Geometry: final body of the model. Coordinates: model frame, mm. A direction names the side the tool comes from. Coordinates: 2 decimals unless noted, no trailing zeros. Write each loop counter-clockwise with the first axis right and the second up, starting at its lowest first coordinate (ties: lowest second). Pieces come first, ordered by that corner, then holes. Notation, with made-up numbers: (70.5, 72) -> (86.5, 72) arc R26 cw to (86.5, 105) -> close; hole circle Ø1 at (4, 69). An arc over 180 degrees is marked (long way). Answer as a JSON object with one key per item and string values. Group by question number.
```python
from build123d import *

# Parameters (mm, degrees)
F3_DEPTH = 16.001
F4_SIZE  = 1


with BuildPart() as f1:
    # F0 (on Front) → F1 (revolve)
    with BuildSketch(Plane.XZ):
        Polygon((-10.15, 13), (-10.15, 0), (0, 0), (0, 1), (-3.15, 1), (-3.15, 8), (-5.15, 8), (-5.15, 16), (-7.15, 16), (-7.15, 13), align=None)
    revolve(axis=Axis((0, 0, -8.6291319943), (0, 0, -1)))

    # F2 (on Top) → F3 (cut, through all)
    with BuildSketch(Plane.XY):
        with BuildLine():
            Line((0, -7.8913969919), (-1.1252094373, -9.3733511499))
            ThreePointArc((-1.1252094373, -9.3733511499), (-1.4401892892, -9.7634180213), (-1.8953023246, -9.9737429991))
            ThreePointArc((-1.8953023246, -9.9737429991), (0, -11.3207029958), (1.8953023246, -9.9737429991))
            ThreePointArc((1.8953023246, -9.9737429991), (1.4401892892, -9.7634180213), (1.1252094373, -9.3733511499))
            Line((1.1252094373, -9.3733511499), (0, -7.8913969919))
        make_face()
        with BuildLine():
            Line((7.5051645318, -2.4385757799), (8.5668778523, -3.9666625671))
            ThreePointArc((8.5668778523, -3.9666625671), (8.8405193649, -4.3867634999), (8.8999126434, -4.8845957104))
            ThreePointArc((8.8999126434, -4.8845957104), (10.7666283532, -3.498289614), (10.0712738989, -1.2795164581))
            ThreePointArc((10.0712738989, -1.2795164581), (9.7306052959, -1.6473606836), (9.2622955289, -1.826387032))
            Line((9.2622955289, -1.826387032), (7.5051645318, -2.4385757799))
        make_face()
        with BuildLine():
            Line((4.6384467718, 6.3842742758), (6.4198311274, 6.9218188615))
            ThreePointArc((6.4198311274, 6.9218188615), (6.9039307349, 7.0522490777), (7.3957508351, 6.9548968288))
            ThreePointArc((7.3957508351, 6.9548968288), (6.6541422665, 9.1586411119), (4.329087255, 9.1829583388))
            ThreePointArc((4.329087255, 9.1829583388), (4.5736555148, 8.7452931271), (4.5992040135, 8.2445818874))
            Line((4.5992040135, 8.2445818874), (4.6384467718, 6.3842742758))
        make_face()
        with BuildLine():
            Line((-4.6384467718, 6.3842742758), (-4.5992040135, 8.2445818874))
            ThreePointArc((-4.5992040135, 8.2445818874), (-4.5736555148, 8.7452931271), (-4.329087255, 9.1829583388))
            ThreePointArc((-4.329087255, 9.1829583388), (-6.6541422665, 9.1586411119), (-7.3957508351, 6.9548968288))
            ThreePointArc((-7.3957508351, 6.9548968288), (-6.9039307349, 7.0522490777), (-6.4198311274, 6.9218188615))
            Line((-6.4198311274, 6.9218188615), (-4.6384467718, 6.3842742758))
        make_face()
        with BuildLine():
            Line((-7.5051645318, -2.4385757799), (-9.2622955289, -1.826387032))
            ThreePointArc((-9.2622955289, -1.826387032), (-9.7306052959, -1.6473606836), (-10.0712738989, -1.2795164581))
            ThreePointArc((-10.0712738989, -1.2795164581), (-10.7666283532, -3.498289614), (-8.8999126434, -4.8845957104))
            ThreePointArc((-8.8999126434, -4.8845957104), (-8.8405193649, -4.3867634999), (-8.5668778523, -3.9666625671))
            Line((-8.5668778523, -3.9666625671), (-7.5051645318, -2.4385757799))
        make_face()
    extrude(amount=F3_DEPTH, mode=Mode.SUBTRACT)

    # F4
    f4_edges = [f1.edges().sort_by_distance(p)[0] for p in [
        (-5.96602, -8.211522, 0),
        (5.96602, -8.211522, 0),
        (9.653224, 3.136522, 0),
        (0, 10.15, 0),
        (-9.653224, 3.136522, 0),
    ]]
    chamfer(f4_edges, length=F4_SIZE)


solid = f1.part
```
Item 1: Set-up query: faces 4 (the flat face through (5.52, 6.65, 6.41)), 5 (the flat face through (-8.371, -2.137, 6.409)), 6 (the flat face through (-0.555, -8.622, 6.409)). Return all of +Z, -Z, +X, -X, +Y, -Y with unobstructed straight access to the full face (end or side cutting, diameter ignored); none if empty.
Item 2: Ray query, L1, parallel to Y at x = 0, z = 13.25; L2, parallel to Z at x = 1.5, y = 3.5; L3, parallel to Y at x = 1.25, z = 6. Return the intervals inside material, ascending. Write a range as [from, to].
Item 3: Mould query, pull axis Y, two halves, no side actions, for faces 1 (the cylindrical face through (0.93, 7.09, 14.48)), 2 (the flat face through (-5.542, 6.657, 6.409)), 3 (the cylindrical face through (-8.84, -4.39, 6.56)). Classes: +Y half, -Y half, draft (parallel to the pull), parting line (faces both ways), or undercut.
Item 4: Contact query for flat-ended pins moving along their axis: pin 1 (2 mm diameter, centred on x = 0.5, z = 5, fed in from -Y); pin 2 (6 mm diameter, centred on x = 0, y = 0, fed in from +Z); pin 3 (1.5 mm diameter, centred on y = 7.5, z = 7.5, fed in from -X). Output: stop coordinate, or through.
Item 5: Section B-B on z = 11.25. Output: boundary loops of the cut face in (x, y).
Item 6: Section A-A on y = 0. Output: boundary loops of the cut face in (x, z).
Answer sheet:
{
 "1": {"face 4": "+Z, -Z, +Y", "face 5": "+Z, -Z, -X", "face 6": "+Z, -Z, -Y"},
 "2": {"L1": "y = [-7.15, -5.15], [5.15, 7.15]", "L2": "z = [0, 8]", "L3": "y = [-9.57, -2.89], [2.89, 10.07]"},
 "3": {"face 1": "parting line", "face 2": "+Y half", "face 3": "undercut"},
 "4": {"pin 1": "stops at y = -9.81", "pin 2": "stops at z = 1", "pin 3": "stops at x = -7.58"},
 "5": {"outline": "(-10.07, -1.28) arc R1.1 ccw to (-9.26, -1.83) -> (-7.51, -2.44) -> (-8.57, -3.97) arc R1.1 ccw to (-8.9, -4.88) arc R10.15 ccw to (-1.89, -9.97) arc R1.1 ccw to (-1.13, -9.37) -> (0, -7.89) -> (1.13, -9.37) arc R1.1 ccw to (1.89, -9.97) arc R10.15 ccw to (8.9, -4.88) arc R1.1 ccw to (8.57, -3.97) -> (7.51, -2.44) -> (9.26, -1.83) arc R1.1 ccw to (10.07, -1.28) arc R10.15 ccw to (7.39, 6.96) arc R1.1 ccw to (6.42, 6.92) -> (4.64, 6.38) -> (4.6, 8.24) arc R1.1 ccw to (4.33, 9.18) arc R10.15 ccw to (-4.33, 9.18) arc R1.1 ccw to (-4.6, 8.24) -> (-4.64, 6.38) -> (-6.42, 6.92) arc R1.1 ccw to (-7.39, 6.96) arc R10.15 ccw to start; hole circle Ø10.3 at (0, 0)"},
 "6": {"outline": "(-10.15, 1) -> (-9.15, 0) -> (9.15, 0) -> (10.15, 1) -> (10.15, 13) -> (7.15, 13) -> (7.15, 16) -> (5.15, 16) -> (5.15, 8) -> (3.15, 8) -> (3.15, 1) -> (-3.15, 1) -> (-3.15, 8) -> (-5.15, 8) -> (-5.15, 16) -> (-7.15, 16) -> (-7.15, 13) -> (-10.15, 13) -> close"}
}
